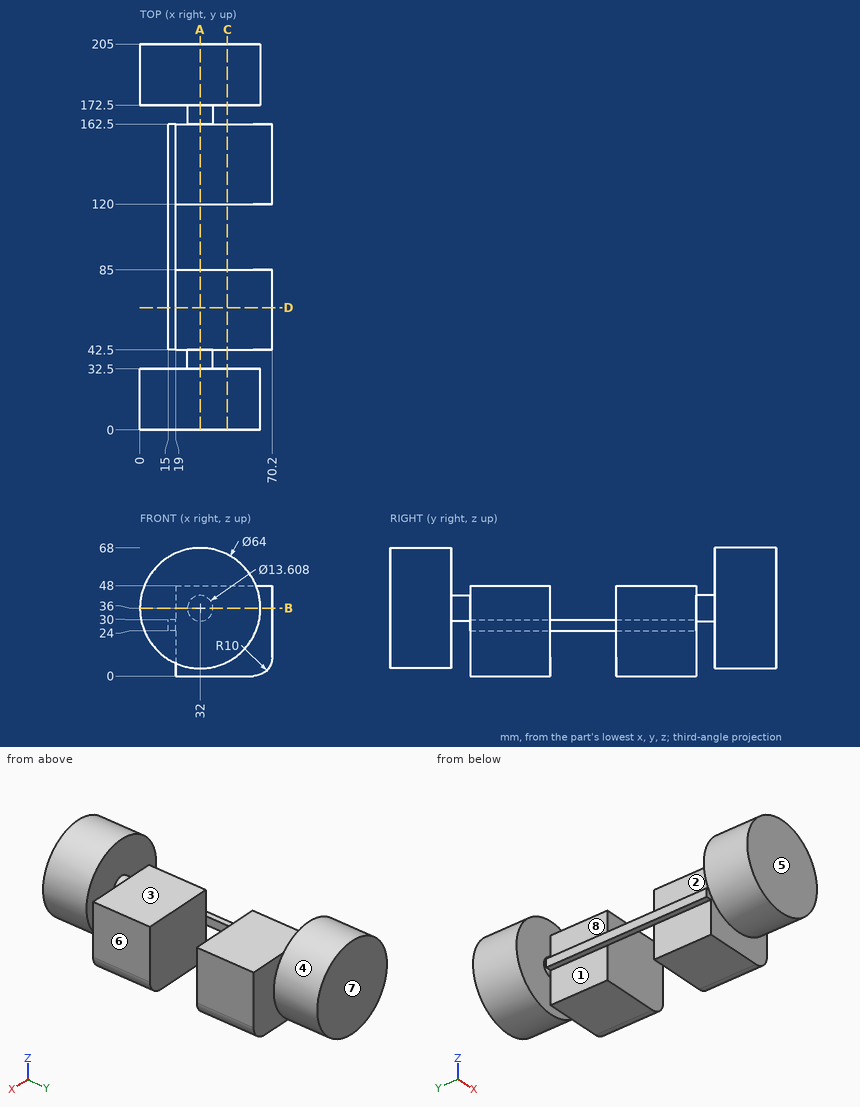
Study the drawing (mm; zero at the part's minimum x, y, z) and answer. A direction names the side the tool comes from. Round coordinates to 2 decimals unless told otherwise and drop trailing zeros. Write each loop counter-clockwise with the first axis right and the second up, starting at its lowest first coordinate (ties: lowest second). Pieces come first, ordered by that corner, then holes.
Q1. Straight lines are drawn through the part: line 1 (Y direction, x = 22.5, z = 37); line 2 (Y direction, x = 28, z = 61); line 3 (Y direction, x = 67, z = 15). For each, find the intervals that lie inside material, in ascending order.
Values:
line 1: y = 0 to 32.5, 42.5 to 85, 120 to 162.5, 172.5 to 205
line 2: y = 0 to 32.5, 172.5 to 205
line 3: y = 42.5 to 85, 120 to 162.5
Q2. Flat-ended cylindrical pins translate along their axes: P1, Ø6, axis at x = 41, y = 121.5, coming from the +Z side; P2, Ø9, axis at y = 135.5, z = 40.5, coming from the -X side; P3, Ø3, axis at y = 96.5, z = 26.5, coming from the +X side. Find the tip coordinate at first contact, or state that the pin passes through.
Values:
P1: stops at z = 48
P2: stops at x = 19
P3: stops at x = 19
Q3. A tool of negligible diameter and unlimited length cuts with its end or side. For the marked faces 1, 2, 3, 4 and 5, from which of +Z, -Z, +X, -X, +Y, -Y can it reach the whole face along a straight path? Write none if from no direction.
Values:
face 1: -Z, -X
face 2: +Z, -X
face 3: +Z, +X, -X
face 4: +Y
face 5: +Z, -Z, +X, -X, -Y
Q4. Find section C-C on x = 46.5. Determine the outline of the cut face in (y, z), and give its area (3 significant figures).
Values:
outline: (0, 7.47) - (32.5, 7.47) - (32.5, 64.53) - (0, 64.53) - close; (42.5, 0) - (85, 0) - (85, 48) - (42.5, 48) - close; (120, 0) - (162.5, 0) - (162.5, 48) - (120, 48) - close; (172.5, 7.47) - (205, 7.47) - (205, 64.53) - (172.5, 64.53) - close
area: 7,790 mm2
Q5. Find section B-B on z = 36. Determine the outline of the cut face in (x, y).
Values:
outline: (0, 0) - (64, 0) - (64, 32.5) - (38.8, 32.5) - (38.8, 42.5) - (70.2, 42.5) - (70.2, 85) - (19, 85) - (19, 42.5) - (25.2, 42.5) - (25.2, 32.5) - (0, 32.5) - close; (0, 172.5) - (25.2, 172.5) - (25.2, 162.5) - (19, 162.5) - (19, 120) - (70.2, 120) - (70.2, 162.5) - (38.8, 162.5) - (38.8, 172.5) - (64, 172.5) - (64, 205) - (0, 205) - close
Q6. The mould has two halves that part along Y. Classify the marked faces 6, 7 and 8: released by +Y, released by -Y, zero draft, split by the parting line, or undercut.
Values:
face 6: zero draft
face 7: released by +Y
face 8: undercut
Q7. Find section A-A on x = 32. Determine the outline of the cut face in (y, z), and give its area (3 significant figures).
Values:
outline: (0, 4) - (32.5, 4) - (32.5, 29.2) - (42.5, 29.2) - (42.5, 0) - (85, 0) - (85, 48) - (42.5, 48) - (42.5, 42.8) - (32.5, 42.8) - (32.5, 68) - (0, 68) - close; (120, 0) - (162.5, 0) - (162.5, 29.2) - (172.5, 29.2) - (172.5, 4) - (205, 4) - (205, 68) - (172.5, 68) - (172.5, 42.8) - (162.5, 42.8) - (162.5, 48) - (120, 48) - close
area: 8,510 mm2
Q8. Find section D-D on y = 65. Determine the outline of the cut face in (x, z), and give its area (3 significant figures).
Values:
outline: (15, 24) - (19, 24) - (19, 0) - (60.2, 0) arc R10 ccw to (70.2, 10) - (70.2, 48) - (19, 48) - (19, 30) - (15, 30) - close
area: 2,460 mm2
